from build123d import *

# Parameters (mm, degrees)
SKETCH_1_R                      = 25
SKETCH_1_R_2                    = 20.1
EXTRUDE_1_DEPTH                 = 10
EXTRUDE_START                   = -10
EXTRUDE_2_DEPTH                 = 10
SKETCH_3_R                      = 9
EXTRUDE_3_DEPTH                 = 6
SKETCH_4_R                      = 2.15
CUT_EXTRUDE_1_DEPTH             = 66.751324099
FILLET_1_R                      = 10
SKETCH_5_R                      = 9
CUT_EXTRUDE_2_DEPTH             = 2.3
CUT_EXTRUDE_START               = -2.3
SKETCH_6_R                      = 9
CUT_EXTRUDE_3_DEPTH             = 2.3
FILLET_START                    = -6
FILLET_2_DEPTH                  = 2.3
FILLET_START_2                  = 3.7
FILLET_2_2_DEPTH                = 2.3
F_3_0MM_1_D                     = 3.5
F_3_0MM_1_DEPTH                 = 4.948493917
F_3_0MM_1_CSINK_D               = 4
F_3_0MM_1_CSINK_ANGLE           = 90
F_3_0MM_1_TIP                   = 1.051506083
F_3_0MM_1_ON_FACE_2_D           = 3.5
F_3_0MM_1_ON_FACE_2_DEPTH       = 4.948493917
F_3_0MM_1_ON_FACE_2_CSINK_D     = 4
F_3_0MM_1_ON_FACE_2_CSINK_ANGLE = 90
F_3_0MM_1_ON_FACE_2_TIP         = 1.051506083
F_3_0MM_1_ON_FACE_3_D           = 3.5
F_3_0MM_1_ON_FACE_3_DEPTH       = 4.948493917
F_3_0MM_1_ON_FACE_3_CSINK_D     = 4
F_3_0MM_1_ON_FACE_3_CSINK_ANGLE = 90
F_3_0MM_1_ON_FACE_3_TIP         = 1.051506083


with BuildPart() as part:
    # 草图1 → 凸台-拉伸1 (new body)
    with BuildSketch(Plane(origin=(0, 0, 0), x_dir=(1, 0, 0), z_dir=(0, 1, 0))):
        with Locations(Location((0, 0, 0), (0, 0, 270))):
            Circle(SKETCH_1_R)
        with Locations(Location((0, 0, 0), (0, 0, 270))):
            Circle(SKETCH_1_R_2, mode=Mode.SUBTRACT)
    extrude(amount=EXTRUDE_1_DEPTH)

    # 草图2 → 凸台-拉伸2 (add)
    with BuildSketch(Plane(origin=(0, 10, 0), x_dir=(1, 0, 0), z_dir=(0, 1, 0)).offset(EXTRUDE_START)):
        with BuildLine():
            Line((-6, 24.269322199), (-6, 40.269322199))
            Line((-6, 40.269322199), (6, 40.269322199))
            Line((6, 40.269322199), (6, 24.269322199))
            ThreePointArc((6, 24.269322199), (0, 25), (-6, 24.269322199))
        make_face()
    extrude(amount=EXTRUDE_2_DEPTH)

    # 草图3 → 凸台-拉伸3 (add, symmetric)
    with BuildSketch(Plane(origin=(0, 0, 0), x_dir=(0, 0, -1), z_dir=(1, 0, 0))):
        with Locations((47.269322199, 5)):
            Circle(SKETCH_3_R)
    extrude(amount=EXTRUDE_3_DEPTH, both=True)

    # 草图4 → 切除-拉伸1 (cut, through all)
    with BuildSketch(Plane(origin=(6, 0, 0), x_dir=(0, 0, -1), z_dir=(1, 0, 0))):
        with Locations((47.269322199, 5)):
            Circle(SKETCH_4_R)
    extrude(amount=-CUT_EXTRUDE_1_DEPTH, mode=Mode.SUBTRACT)

    # 圆角1
    fillet_1_edges = [part.edges().sort_by_distance(p)[0] for p in [
        (6, 5, -24.269322199),
        (-6, 5, -24.269322199),
        (0, 10, -39.786007425),
        (0, 0, -39.786007425),
    ]]
    fillet(fillet_1_edges, radius=FILLET_1_R)

    # 草图5 → 切除-拉伸2 (cut)
    with BuildSketch(Plane(origin=(6, 0, 0), x_dir=(0, 0, -1), z_dir=(1, 0, 0))):
        with Locations((47.269322199, 5)):
            Circle(SKETCH_5_R)
    extrude(amount=-CUT_EXTRUDE_2_DEPTH, mode=Mode.SUBTRACT)

    # 草图6 → 切除-拉伸3 (cut)
    with BuildSketch(Plane.ZY.offset(6).offset(CUT_EXTRUDE_START)):
        with Locations((-47.269322199, 5)):
            Circle(SKETCH_6_R)
    extrude(amount=CUT_EXTRUDE_3_DEPTH, mode=Mode.SUBTRACT)

    # 圆角2: read off the stored shape, not the designer's step
    # 圆角2 outline → 圆角2 (cut)
    with BuildSketch(Plane.YZ.offset(FILLET_START)):
        with BuildLine():
            ThreePointArc((10.29326278, -38.011426009), (9.953936392, -39.027326957), (8.890330152, -39.153576312))
            ThreePointArc((8.890330152, -39.153576312), (10.648449114, -40.262538157), (12.105263158, -41.745262509))
            ThreePointArc((12.105263158, -41.745262509), (11.003425316, -39.973382673), (10.29326278, -38.011426009))
        make_face()
        with BuildLine():
            ThreePointArc((-2.105263158, -41.745262509), (-0.648449114, -40.262538157), (1.109669848, -39.153576312))
            ThreePointArc((1.109669848, -39.153576312), (0.046063608, -39.027326957), (-0.29326278, -38.011426009))
            ThreePointArc((-0.29326278, -38.011426009), (-1.003425316, -39.973382673), (-2.105263158, -41.745262509))
        make_face()
    extrude(amount=FILLET_2_DEPTH, mode=Mode.SUBTRACT)

    # Fillet 2 2 outline → Fillet 2 2 (cut)
    with BuildSketch(Plane.YZ.offset(FILLET_START_2)):
        with BuildLine():
            ThreePointArc((10.29326278, -38.011426009), (9.953936392, -39.027326957), (8.890330152, -39.153576312))
            ThreePointArc((8.890330152, -39.153576312), (10.648449114, -40.262538157), (12.105263158, -41.745262509))
            ThreePointArc((12.105263158, -41.745262509), (11.003425316, -39.973382673), (10.29326278, -38.011426009))
        make_face()
        with BuildLine():
            ThreePointArc((-2.105263158, -41.745262509), (-0.648449114, -40.262538157), (1.109669848, -39.153576312))
            ThreePointArc((1.109669848, -39.153576312), (0.046063608, -39.027326957), (-0.29326278, -38.011426009))
            ThreePointArc((-0.29326278, -38.011426009), (-1.003425316, -39.973382673), (-2.105263158, -41.745262509))
        make_face()
    extrude(amount=FILLET_2_2_DEPTH, mode=Mode.SUBTRACT)

    # Ø3.0mm 暗销孔1
    with Locations(Plane(origin=(0, 5, 25), x_dir=(1, 0, 0), z_dir=(0, 0, 1))):
        with Locations((0, 0)):
            CounterSinkHole(F_3_0MM_1_D / 2, F_3_0MM_1_CSINK_D / 2, depth=F_3_0MM_1_DEPTH, counter_sink_angle=F_3_0MM_1_CSINK_ANGLE)
            with Locations((0, 0, -(F_3_0MM_1_DEPTH + F_3_0MM_1_TIP / 2))):  # 118° drill point
                Cone(0, F_3_0MM_1_D / 2, F_3_0MM_1_TIP, mode=Mode.SUBTRACT)

    # Ø3.0mm 暗销孔1 on face 2
    with Locations(Plane(origin=(-21.650635095, 5, -12.5), x_dir=(0.500000174844, 0, -0.866025302838), z_dir=(-0.866025302838, 0, -0.500000174844))):
        with Locations((0, 0)):
            CounterSinkHole(F_3_0MM_1_ON_FACE_2_D / 2, F_3_0MM_1_ON_FACE_2_CSINK_D / 2, depth=F_3_0MM_1_ON_FACE_2_DEPTH, counter_sink_angle=F_3_0MM_1_ON_FACE_2_CSINK_ANGLE)
            with Locations((0, 0, -(F_3_0MM_1_ON_FACE_2_DEPTH + F_3_0MM_1_ON_FACE_2_TIP / 2))):  # 118° drill point
                Cone(0, F_3_0MM_1_ON_FACE_2_D / 2, F_3_0MM_1_ON_FACE_2_TIP, mode=Mode.SUBTRACT)

    # Ø3.0mm 暗销孔1 on face 3
    with Locations(Plane(origin=(21.650635095, 5, -12.5), x_dir=(0.500000174844, 0, 0.866025302838), z_dir=(0.866025302838, 0, -0.500000174844))):
        with Locations((0, 0)):
            CounterSinkHole(F_3_0MM_1_ON_FACE_3_D / 2, F_3_0MM_1_ON_FACE_3_CSINK_D / 2, depth=F_3_0MM_1_ON_FACE_3_DEPTH, counter_sink_angle=F_3_0MM_1_ON_FACE_3_CSINK_ANGLE)
            with Locations((0, 0, -(F_3_0MM_1_ON_FACE_3_DEPTH + F_3_0MM_1_ON_FACE_3_TIP / 2))):  # 118° drill point
                Cone(0, F_3_0MM_1_ON_FACE_3_D / 2, F_3_0MM_1_ON_FACE_3_TIP, mode=Mode.SUBTRACT)


solid = part.part
Input: part model. Units: mm. Frame: model coordinates. A direction names the side the tool comes from. Give positions to 0.01 mm unless a question says otherwise; leave off trailing zeros. Order: outer loops, then holes, each group sorted by start corner. A loop starts at its lowest first (then second) coordinate and runs counter-clockwise, first axis right, second up. Notation, with made-up numbers: M -38.5,25 L 13.5,25 A9 cw 13.5,38 Z; hole C 36.5,-0.5 d10. An arc over 180 degrees is marked long. Answer as a JSON object with one key per item and string values.
1. Cut plane C-C, the plane y = 5. State how many separate pieces and enclosed holes the cut face has, and give its area (3 significant figures).
Result sheet:
{"separate pieces": "4", "enclosed holes": "0", "area": "921 mm²"}
2. Cut plane B-B, the plane z = 0. Output: boundary loops of the cut face in (x, y).
Result sheet:
{"outline": "M -25,0 L -20.1,0 L -20.1,10 L -25,10 Z; M 20.1,0 L 25,0 L 25,10 L 20.1,10 Z"}
3. Cut plane A-A, the plane x = 0. Output: boundary loops of the cut face in (y, z), and give its area (3 significant figures).
Result sheet:
{"outline": "M -2.11,-41.75 A9 ccw long 12.11,-41.75 A10 cw 10,-35.61 L 10,-20.1 L 0,-20.1 L 0,-35.61 A10 cw Z; M 0,20.1 L 3.25,20.1 L 3.25,24.75 L 3,25 L 0,25 Z; M 6.75,20.1 L 10,20.1 L 10,25 L 7,25 L 6.75,24.75 Z; hole C 5,-47.27 d4.3", "area": "462 mm²"}
4. Pull-direction query (Z, two-part tool) for faces 1 (the cylindrical face through (0.08, 10.34, -38.19)), 2 (the cylindrical face through (7.425, 5.07, -25.985)), 3 (the cylindrical face through (19.56, 6.71, -10.86)); classes: +Z half, -Z half, draft (parallel to the pull), parting line (faces both ways), or undercut.
Result sheet:
{"face 1": "+Z half", "face 2": "-Z half", "face 3": "undercut"}
5. First-contact query: P1, Ø1.5, axis at x = 17.5, y = 7.5, coming from the -Z side; P2, Ø8, axis at y = 6.5, z = 7.5, coming from the -X side; P3, Ø4, axis at y = 6, z = -37, coming from the +X side; P4, Ø1, axis at x = 16, z = -9.5, coming from the -Y side. Flat tips, straight axial feed; report the tip coordinate or a pass-through.
Result sheet:
{"P1": "z = -18.56", "P2": "x = -24.75", "P3": "x = 6", "P4": "through"}
6. Reachability of faces 4 (the cylindrical face through (-4.83, 4.94, -38.27)), 5 (the flat face through (6, 5, -35)), 6 (the cylindrical face through (4.87, 5.06, -38.27)), 7 (the cylindrical face through (0.38, 3.29, 22.37)) from +Z, -Z, +X, -X, +Y, -Y: full face, straight path, thin tool, end or side. Return the list, or none.
Result sheet:
{"face 4": "-Z, -X", "face 5": "-Z, +X, +Y, -Y", "face 6": "-Z, +X", "face 7": "+Z"}
7. Ray query, line 1 (Y direction, x = -6, z = -27); line 2 (X direction, y = -0.5, z = -40); line 3 (X direction, y = 5.5, z = 0). Return the intervals inside material, ascending. Write a range as [from, to].
Result sheet:
{"line 1": "[0, 10]", "line 2": "[-3.7, 3.7]", "line 3": "[-25, -20.1], [20.1, 25]"}
8. Cut plane D-D, the plane z = -16. Output: boundary loops of the cut face in (x, y), and give its area (3 significant figures).
Result sheet:
{"outline": "M -19.21,0 L -12.17,0 L -12.17,10 L -19.21,10 Z; M 12.17,0 L 19.21,0 L 19.21,10 L 12.17,10 Z", "area": "141 mm²"}
